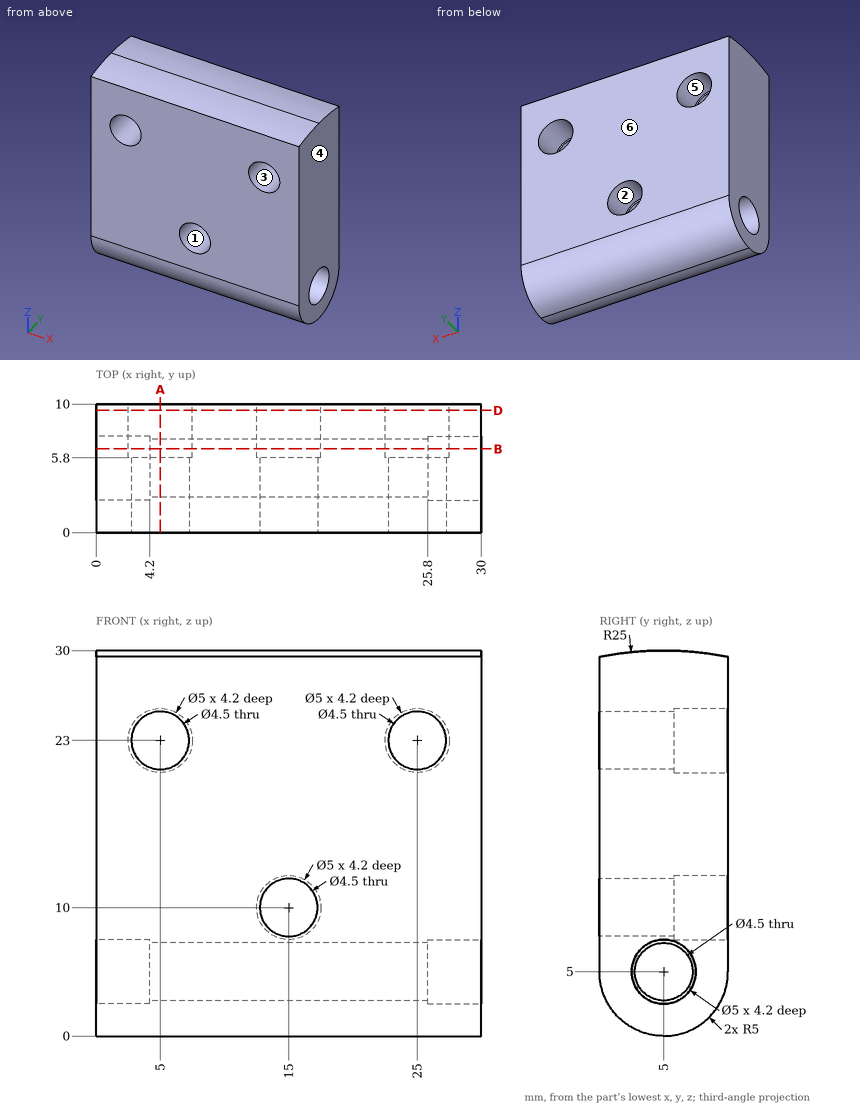
Input: dimensioned drawing with shaded views. Units: mm. Origin: part minimum x, y, z. A direction names the side the tool comes from. Round coordinates to 2 decimals unless told otherwise and drop trailing zeros. Loops run counter-clockwise (first coordinate to the right, second up) from the corner with the lowest first, then second, coordinate; pieces in that order, holes last. Notation, with made-up numbers: (-10.5, 26.5) -> (19.5, 26.5) arc R29 cw to (19.5, 55.5) -> close; hole circle Ø2 at (-14.75, -10.5). An arc over 180 degrees is marked (long way). Answer as a JSON object with one key per item and string values. Group by question number.
Q1. Section query B-B (y = 6.5). Output: boundary loops of the cut face in (x, z) (3 decimals).
Q2. Ray query, line 1 (X direction, y = 2.9, z = 23); line 2 (X direction, y = 8.4, z = 23); line 3 (Y direction, x = 1.6, z = 5). Return the intervals inside material, ascending. Write a range as from..to.
Q3. Mould query, pull axis X, two halves, no side actions, for the marked faces 3, 4, 5 and 6. Classes: pulls with the +X half, pulls with the -X half, needs draft (parallel to the pull), parting line crosses it, or undercut.
Q4. Section query A-A (x = 5). State how many separate pieces and enclosed holes the cut face has, plus the area to 3 significant figures.
Q5. Access query for the marked faces 1 and 2. Directions: +Z, -Z, +X, -X, +Y, -Y. A direction counts if a zero-diameter tool reaches every point of the face in a straight line with its end or side. Return the directions, or none.
Q6. Section query D-D (y = 9.5). Output: boundary loops of the cut face in (x, z).
Q7. Contact query for flat-ended pins moving along their axis: P1, Ø6, axis at x = 15, z = 10, coming from the +Y side; P2, Ø1.5, axis at x = 16.5, y = 6, coming from the -Z side. Output: stop coordinate, or through.
Completed:
{
 "1": {"outline": "(0, 0.23) -> (30, 0.23) -> (30, 3) -> (25.8, 3) -> (25.8, 3.323) -> (4.2, 3.323) -> (4.2, 3) -> (0, 3) -> close; (0, 7) -> (4.2, 7) -> (4.2, 6.677) -> (25.8, 6.677) -> (25.8, 7) -> (30, 7) -> (30, 29.955) -> (0, 29.955) -> close; hole circle Ø5 at (5, 23); hole circle Ø5 at (15, 10); hole circle Ø5 at (25, 23)"},
 "2": {"line 1": "0..2.75, 7.25..22.75, 27.25..30", "line 2": "0..2.5, 7.5..22.5, 27.5..30", "line 3": "0..2.5, 7.5..10"},
 "3": {"face 3": "undercut", "face 4": "pulls with the +X half", "face 5": "undercut", "face 6": "needs draft"},
 "4": {"separate pieces": "2", "enclosed holes": "1", "area": "225 mm²"},
 "5": {"face 1": "+Y, -Y", "face 2": "+Y"},
 "6": {"outline": "(0, 2.82) -> (30, 2.82) -> (30, 29.59) -> (0, 29.59) -> close; hole circle Ø5 at (5, 23); hole circle Ø5 at (15, 10); hole circle Ø5 at (25, 23)"},
 "7": {"P1": "y = 10", "P2": "z = 0.01"}
}
